Verification items for this drawing (mm, ordinates from the low corner). Round coordinates to 2 decimals unless told otherwise and drop trailing zeros. Order: outer loops, then holes, each group sorted by start corner. A loop starts at its lowest first (then second) coordinate and runs counter-clockwise, first axis right, second up.
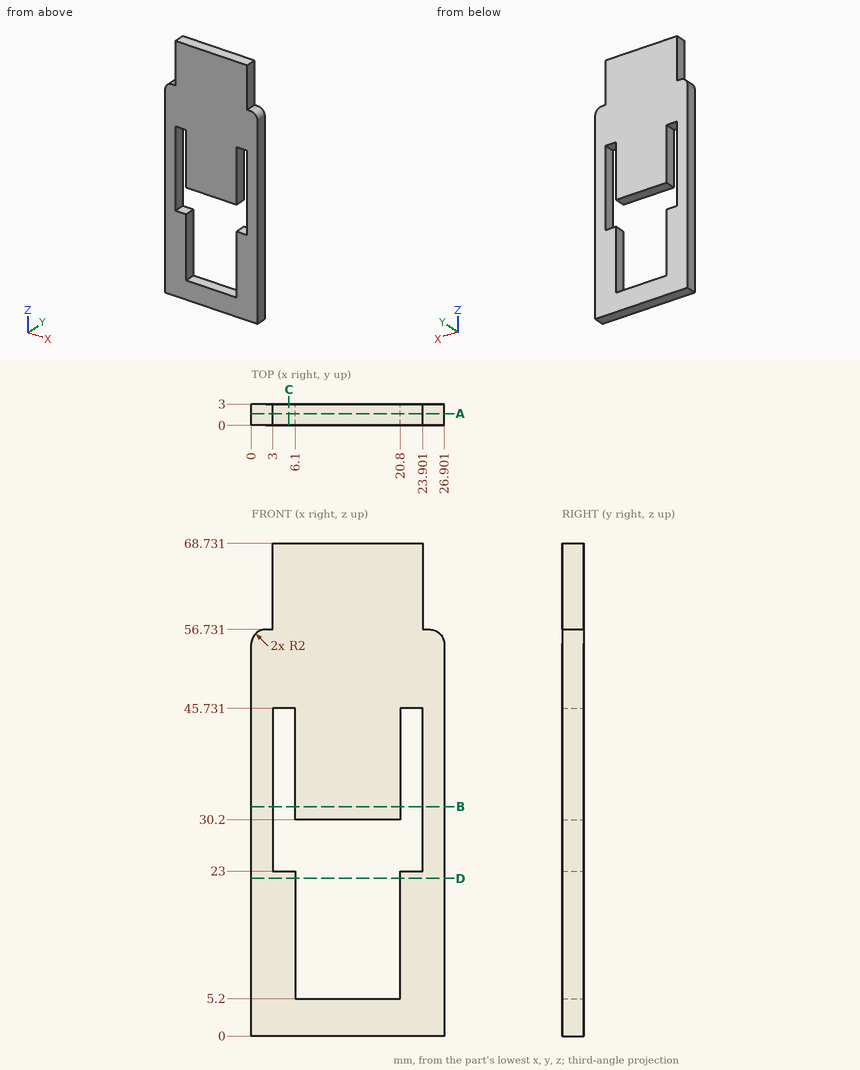
Item 1: Scan lines: line 1 along X through (y, z) = (0.95, 38.5); line 2 along X through (y, z) = (0.35, 24); line 3 along Z through (x, y) = (5.75, 0.7). Record each from-to range of solid material in increasing order.
Answer:
line 1: x = 0 to 3, 6.1 to 20.8, 23.9 to 26.9
line 2: x = 0 to 3, 23.9 to 26.9
line 3: z = 0 to 23, 45.73 to 68.73
Item 2: Go/stop test with a flat-tipped pin: P1, Ø0.5, axis at x = 24.5, y = 1, coming from the +Z side. Record where the tip stops, or that it passes through.
Answer:
P1: stops at z = 56.73
Item 3: Sectioned sample at B-B (z = 32). Record the cut outline in (x, y).
Answer:
outline: (0, 0) - (3, 0) - (3, 3) - (0, 3) - close; (6.1, 0) - (20.8, 0) - (20.8, 3) - (6.1, 3) - close; (23.9, 0) - (26.9, 0) - (26.9, 3) - (23.9, 3) - close
Item 4: Sectioned sample at C-C (x = 5.25). Record the cut outline in (y, z), and give its area (3 significant figures).
Answer:
outline: (0, 0) - (3, 0) - (3, 23) - (0, 23) - close; (0, 45.73) - (3, 45.73) - (3, 68.73) - (0, 68.73) - close
area: 138 mm2
Item 5: Sectioned sample at A-A (y = 1.65). Record the cut outline in (x, z).
Answer:
outline: (0, 0) - (26.9, 0) - (26.9, 54.73) arc R2 ccw to (24.9, 56.73) - (23.9, 56.73) - (23.9, 68.73) - (3, 68.73) - (3, 56.73) - (2, 56.73) arc R2 ccw to (0, 54.73) - close; hole (3, 23) - (6.1, 23) - (6.1, 5.2) - (20.8, 5.2) - (20.8, 23) - (23.9, 23) - (23.9, 45.73) - (20.8, 45.73) - (20.8, 30.2) - (6.1, 30.2) - (6.1, 45.73) - (3, 45.73) - close
Item 6: Sectioned sample at D-D (z = 22). Record the cut outline in (x, y), and give its area (3 significant figures).
Answer:
outline: (0, 0) - (6.1, 0) - (6.1, 3) - (0, 3) - close; (20.8, 0) - (26.9, 0) - (26.9, 3) - (20.8, 3) - close
area: 36.6 mm2
